Part model, mm, in its own coordinate system. Coordinates: 2 decimals unless noted, no trailing zeros. Order: outer loops, then holes, each group sorted by start corner. A loop starts at its lowest first (then second) coordinate and runs counter-clockwise, first axis right, second up. Notation, with made-up numbers: (58.5, 83) - (99.5, 83) arc R17 cw to (99.5, 107) - close; hole circle Ø10 at (49, 30). An arc over 180 degrees is marked (long way). Use a Markdown table: item, result. Add a question column.
1) Saw through at B-B on x = -0.75. List the corners of the cut face in (y, z), then the cut area to 4 significant figures.
2) Drop flat-ended pins along their axis: P1, Ø1, axis at y = -4.5, z = 243, coming from the +X side; P2, Ø1, axis at x = -7, z = 88, coming from the +Y side. Give the stop position or say it passes through.
3) Wall check: L1, parallel to Y at x = -17, z = 45; L2, parallel to Y at x = -16.45, z = 90; L3, parallel to Y at x = -6, z = 171.5. Give the ranges that are in metal, low to high. Write a range as [from, to].
4) Saw through at A-A on z = 56. List the corners of the cut face in (x, y).
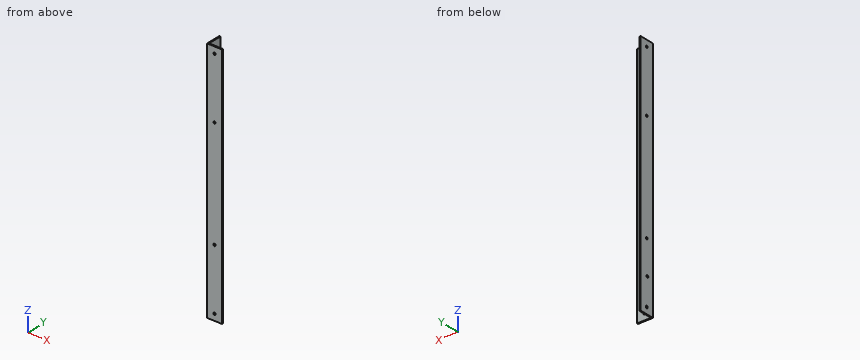
```python
from build123d import *

# Parameters (mm, degrees)
EXTRUSION1_DEPTH = 325
ESQUISSE2_R      = 1.5
EXTRUSION2_DEPTH = 300
ESQUISSE3_R      = 1.5
EXTRUSION3_DEPTH = 300


with BuildPart() as part:
    # Esquisse1 → Extrusion1 (new body)
    with BuildSketch(Plane.XY):
        Polygon((-17.43168638, 4.773368421), (-17.43168638, -15.226631579), (2.56831362, -15.226631579), (2.56831362, -13.726631579), (-15.93168638, -13.726631579), (-15.93168638, 4.773368421), align=None)
    extrude(amount=EXTRUSION1_DEPTH)

    # Esquisse2 → Extrusion2 (cut)
    with BuildSketch(Plane(origin=(0, -13.726631579, 0), x_dir=(-1, 0, 0), z_dir=(0, 1, 0))):
        with Locations((7.43168638, 8.5)):
            Circle(ESQUISSE2_R)
        with Locations((7.43168638, 316.5)):
            Circle(ESQUISSE2_R)
        with Locations((7.43168638, 235)):
            Circle(ESQUISSE2_R)
        with Locations((7.43168638, 90)):
            Circle(ESQUISSE2_R)
    extrude(amount=-EXTRUSION2_DEPTH, mode=Mode.SUBTRACT)

    # Esquisse3 → Extrusion3 (cut)
    with BuildSketch(Plane(origin=(-15.93168638, 0, 0), x_dir=(0, 0, -1), z_dir=(1, 0, 0))):
        with Locations((-316.5, -5.226631579)):
            Circle(ESQUISSE3_R)
        with Locations((-8.5, -5.226631579)):
            Circle(ESQUISSE3_R)
        with Locations((-235, -5.226631579)):
            Circle(ESQUISSE3_R)
        with Locations((-90, -5.226631579)):
            Circle(ESQUISSE3_R)
        with Locations((-45, -6.226631579)):
            Circle(ESQUISSE3_R)
    extrude(amount=-EXTRUSION3_DEPTH, mode=Mode.SUBTRACT)


solid = part.part
```
Results are:
| question | item | result |
|---|---|---|
| 1 | outline | (-15.23, 0) - (-13.73, 0) - (-13.73, 325) - (-15.23, 325) - close |
| 1 | area | 487.5 mm2 |
| 2 | P1 | x = -15.93 |
| 2 | P2 | y = -13.73 |
| 3 | L1 | [-15.23, -7.73], [-4.73, 4.77] |
| 3 | L2 | [-15.23, -6.73], [-3.73, 4.77] |
| 3 | L3 | [-15.23, -13.73] |
| 4 | outline | (-17.43, -15.23) - (2.57, -15.23) - (2.57, -13.73) - (-15.93, -13.73) - (-15.93, 4.77) - (-17.43, 4.77) - close |
